The listing builds one solid part. Answer for the finished solid, in the listing's coordinates (mm). Coordinates: 2 decimals unless noted, no trailing zeros. Write each loop counter-clockwise with the first axis right and the second up, starting at its lowest first coordinate (ties: lowest second). Pieces come first, ordered by that corner, then holes.
Autodesk Inventor part; units mm, degrees
ref_plane "YZ Plane" through (0, 0, 0) normal (1, 0, 0) x (0, 1, 0)
ref_plane "XZ Plane" through (0, 0, 0) normal (0, 1, 0) x (-1, 0, 0)
ref_plane "XY Plane" through (0, 0, 0) normal (0, 0, 1) x (1, 0, 0)
sketch "Sketch1" plane through (0, 0, 0) normal (0, 1, 0) x (-1, 0, 0)
  line L0 (0, 0) -> (101.6, 0)
  line L1 (101.6, 0) -> (101.6, -101.6)
  line L2 (101.6, -101.6) -> (0, -101.6)
  line L3 (0, -101.6) -> (0, 0)
  line L4 (4.7625, -96.8375) -> (96.8375, -96.8375)
  line L5 (96.8375, -96.8375) -> (96.8375, -4.7625)
  line L6 (96.8375, -4.7625) -> (4.7625, -4.7625)
  line L7 (4.7625, -4.7625) -> (4.7625, -96.8375)
  line L8 (96.8375, -4.7625) -> (4.7625, -96.8375) construction
  circle A0 centre (50.8, -50.8) radius 2.5527
  circle A1 centre (50.8, -50.8) radius 5.7277
  line L9 (54.850096, -46.749904) -> (94.143423, -7.456577) construction
  line L10 (58.442198, -46.749904) -> (94.143423, -11.048679)
  line L11 (90.551321, -7.456577) -> (54.850096, -43.157802)
  arc A2 (54.850096, -43.157802) -> (58.442198, -46.749904) centre (56.646147, -44.953853) ccw
  arc A3 (94.143423, -11.048679) -> (90.551321, -7.456577) centre (92.347372, -9.252628) ccw
  line L12 (46.749904, -43.157802) -> (11.048679, -7.456577)
  arc A4 (43.157802, -46.749904) -> (46.749904, -43.157802) centre (44.953853, -44.953853) ccw
  line L13 (7.456577, -11.048679) -> (43.157802, -46.749904)
  arc A5 (11.048679, -7.456577) -> (7.456577, -11.048679) centre (9.252628, -9.252628) ccw
  line L14 (43.157802, -54.850096) -> (7.456577, -90.551321)
  arc A6 (46.749904, -58.442198) -> (43.157802, -54.850096) centre (44.953853, -56.646147) ccw
  line L15 (11.048679, -94.143423) -> (46.749904, -58.442198)
  arc A7 (7.456577, -90.551321) -> (11.048679, -94.143423) centre (9.252628, -92.347372) ccw
  line L16 (54.850096, -58.442198) -> (90.551321, -94.143423)
  arc A8 (58.442198, -54.850096) -> (54.850096, -58.442198) centre (56.646147, -56.646147) ccw
  line L17 (94.143423, -90.551321) -> (58.442198, -54.850096)
  arc A9 (90.551321, -94.143423) -> (94.143423, -90.551321) centre (92.347372, -92.347372) ccw
  point P0 (0, -50.8)
  point P1 (74.496759, -27.103241)
  dimension "d0" = 101.6
  dimension "d1" = 101.6
  dimension "d2" = 4.7625
  dimension "d33" = 5.1054
  dimension "d34" = 3.175
  dimension "d35" = 5.08
  dimension "d36" = 6.35
  dimension "d39" = 360
extrude "Extrusion1" add sketch "Sketch1" along normal blind 6.35 contours L0 L1 L2 L3 | L7 L6 L5 L4 | A1
sketch "Sketch2" plane through (0, 6.35, 0) normal (0, 1, 0) x (1, 0, 0)
  line L0 (0, 101.6) -> (-101.6, 101.6)
  line L1 (-101.6, 101.6) -> (-101.6, 0)
  line L2 (-101.6, 0) -> (0, 0)
  line L3 (0, 0) -> (0, 101.6)
  circle A0 centre (-99.21875, 99.21875) radius 0.79375
  circle A1 centre (-99.21875, 2.38125) radius 0.79375
  circle A2 centre (-2.38125, 99.21875) radius 0.79375
  circle A3 centre (-2.38125, 2.38125) radius 0.79375
  dimension "d20" = 1.5875
  dimension "d21" = 2.38125
  dimension "d22" = 2.38125
  dimension "d25" = 96.8375
  dimension "d28" = 96.8375
extrude "Extrusion2" cut sketch "Sketch2" against normal blind 6.35 contours A0 | A1 | A2 | A3
sketch "Sketch3" plane through (0, 6.35, 0) normal (0, 1, 0) x (1, 0, 0)
  circle A0 centre (-99.21875, 99.21875) radius 0.79375
  circle A1 centre (-99.21875, 2.38125) radius 0.79375
  circle A2 centre (-2.38125, 99.21875) radius 0.79375
  circle A3 centre (-2.38125, 2.38125) radius 0.79375
  line L0 (0, 101.6) -> (-101.6, 101.6)
  line L1 (-101.6, 101.6) -> (-101.6, 0)
  line L2 (-101.6, 0) -> (0, 0)
  line L3 (0, 0) -> (0, 101.6)
  arc A4 (-58.442198, 54.850096) -> (-54.850096, 58.442198) centre (-56.646147, 56.646147) ccw
  line L4 (-58.442198, 54.850096) -> (-94.143423, 90.551321)
  arc A5 (-90.551321, 94.143423) -> (-94.143423, 90.551321) centre (-92.347372, 92.347372) ccw
  line L5 (-90.551321, 94.143423) -> (-54.850096, 58.442198)
  circle A6 centre (-50.8, 50.8) radius 2.5527
  arc A7 (-46.749904, 58.442198) -> (-43.157802, 54.850096) centre (-44.953853, 56.646147) ccw
  line L6 (-46.749904, 58.442198) -> (-11.048679, 94.143423)
  arc A8 (-7.456577, 90.551321) -> (-11.048679, 94.143423) centre (-9.252628, 92.347372) ccw
  line L7 (-7.456577, 90.551321) -> (-43.157802, 54.850096)
  arc A9 (-43.157802, 46.749904) -> (-46.749904, 43.157802) centre (-44.953853, 44.953853) ccw
  line L8 (-43.157802, 46.749904) -> (-7.456577, 11.048679)
  arc A10 (-11.048679, 7.456577) -> (-7.456577, 11.048679) centre (-9.252628, 9.252628) ccw
  line L9 (-11.048679, 7.456577) -> (-46.749904, 43.157802)
  arc A11 (-54.850096, 43.157802) -> (-58.442198, 46.749904) centre (-56.646147, 44.953853) ccw
  line L10 (-54.850096, 43.157802) -> (-90.551321, 7.456577)
  arc A12 (-94.143423, 11.048679) -> (-90.551321, 7.456577) centre (-92.347372, 9.252628) ccw
  line L11 (-94.143423, 11.048679) -> (-58.442198, 46.749904)
sketch "Sketch4" plane through (0, 6.35, 0) normal (0, 1, 0) x (1, 0, 0)
  circle A0 centre (-99.21875, 99.21875) radius 0.79375
  circle A1 centre (-99.21875, 2.38125) radius 0.79375
  circle A2 centre (-2.38125, 99.21875) radius 0.79375
  circle A3 centre (-2.38125, 2.38125) radius 0.79375
  line L0 (0, 101.6) -> (-101.6, 101.6)
  line L1 (-101.6, 101.6) -> (-101.6, 0)
  line L2 (-101.6, 0) -> (0, 0)
  line L3 (0, 0) -> (0, 101.6)
  arc A4 (-58.442198, 54.850096) -> (-54.850096, 58.442198) centre (-56.646147, 56.646147) ccw
  line L4 (-58.442198, 54.850096) -> (-94.143423, 90.551321)
  arc A5 (-90.551321, 94.143423) -> (-94.143423, 90.551321) centre (-92.347372, 92.347372) ccw
  line L5 (-90.551321, 94.143423) -> (-54.850096, 58.442198)
  circle A6 centre (-50.8, 50.8) radius 2.5527
  arc A7 (-46.749904, 58.442198) -> (-43.157802, 54.850096) centre (-44.953853, 56.646147) ccw
  line L6 (-46.749904, 58.442198) -> (-11.048679, 94.143423)
  arc A8 (-7.456577, 90.551321) -> (-11.048679, 94.143423) centre (-9.252628, 92.347372) ccw
  line L7 (-7.456577, 90.551321) -> (-43.157802, 54.850096)
  arc A9 (-43.157802, 46.749904) -> (-46.749904, 43.157802) centre (-44.953853, 44.953853) ccw
  line L8 (-43.157802, 46.749904) -> (-7.456577, 11.048679)
  arc A10 (-11.048679, 7.456577) -> (-7.456577, 11.048679) centre (-9.252628, 9.252628) ccw
  line L9 (-11.048679, 7.456577) -> (-46.749904, 43.157802)
  arc A11 (-54.850096, 43.157802) -> (-58.442198, 46.749904) centre (-56.646147, 44.953853) ccw
  line L10 (-54.850096, 43.157802) -> (-90.551321, 7.456577)
  arc A12 (-94.143423, 11.048679) -> (-90.551321, 7.456577) centre (-92.347372, 9.252628) ccw
  line L11 (-94.143423, 11.048679) -> (-58.442198, 46.749904)
  circle A13 centre (-36.53596, 36.53596) radius 2.159
  line L12 (-44.953853, 44.953853) -> (-9.252628, 9.252628) construction
  circle A14 centre (-50.8, 50.8) radius 25.4
  line L13 (-45.068826, 32.632552) -> (-56.531174, 68.967448) construction
  circle A15 centre (-45.068826, 32.632552) radius 2.159 construction
  circle A16 centre (-56.531174, 68.967448) radius 2.159 construction
  line L14 (-56.531174, 68.967448) -> (-36.53596, 36.53596) construction
  dimension "d41" = 4.318
  dimension "d42" = 50.8
  dimension "d43" = 4.318
  dimension "d44" = 4.318
  dimension "d45" = 38.1
  dimension "d46" = 38.1
ref_plane "Work Plane1" through (-56.646147, 0, -44.953853) normal (0.7071068, 0, 0.7071068) x (0.7071068, 0, -0.7071068)
properties part number "Layer 5"
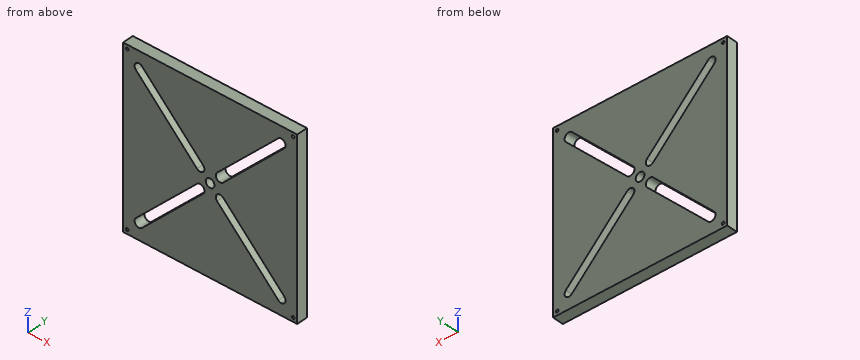
1. Section C-C on y = 3.25 is taken. State how many separate pieces and enclosed holes the cut face has, then the cut area to 3 significant figures.
Results found:
separate pieces: 1
enclosed holes: 9
area: 9,190 mm2
2. Flat-ended cylindrical pins translate along their axes: P1, Ø10, axis at x = -65.5, z = -28.5, coming from the -Y side; P2, Ø4.5, axis at x = -50.8, z = -50.8, coming from the +Y side. Find the tip coordinate at first contact, or state that the pin passes through.
Results found:
P1: stops at y = 0
P2: passes through
3. Find the intervals of material crossed by L1, parallel to Z at x = -50.8, y = 2; L2, parallel to X at y = 2.25, z = -64.5; L3, parallel to Z at x = -18, y = 0.5, in increasing order.
Results found:
L1: z = -101.6 to -53.35, -48.25 to 0
L2: x = -101.6 to -68.09, -60.91 to -40.69, -33.51 to 0
L3: z = -101.6 to -87.19, -80.01 to -21.59, -14.41 to 0
4. Section D-D on z = -72.5 is taken. Give the vertices of the cut face in (x, y).
Results found:
outline: (-101.6, 0) - (-76.09, 0) - (-76.09, 6.35) - (-101.6, 6.35) - close; (-68.91, 0) - (-32.69, 0) - (-32.69, 6.35) - (-68.91, 6.35) - close; (-25.51, 0) - (0, 0) - (0, 6.35) - (-25.51, 6.35) - close
5. Section B-B on x = -50.8 is taken. Give the vertices of the cut face in (y, z), then the cut area to 3 significant figures.
Results found:
outline: (0, -101.6) - (6.35, -101.6) - (6.35, -53.35) - (0, -53.35) - close; (0, -48.25) - (6.35, -48.25) - (6.35, 0) - (0, 0) - close
area: 613 mm2
6. Section A-A on z = -50.8 is taken. Give the vertices of the cut face in (x, y), then the cut area to 3 significant figures.
Results found:
outline: (-101.6, 0) - (-53.35, 0) - (-53.35, 6.35) - (-101.6, 6.35) - close; (-48.25, 0) - (0, 0) - (0, 6.35) - (-48.25, 6.35) - close
area: 613 mm2
